The listing builds one solid part. Answer for the finished solid, in the listing's coordinates (mm). Face numbers are marked on the shaded views. A direction names the side the tool comes from. Round coordinates to 2 decimals unless told otherwise and drop trailing zeros. Loops run counter-clockwise (first coordinate to the right, second up) from the corner with the lowest first, then second, coordinate; pieces in that order, holes last. Notation, with made-up numbers: (68.25, -6) -> (113.25, -6) arc R24 ccw to (113.25, 24) -> close; hole circle Ø6 at (-12, 74). An arc over 180 degrees is marked (long way). Answer in a Markdown table with one row per item. Add a question column.
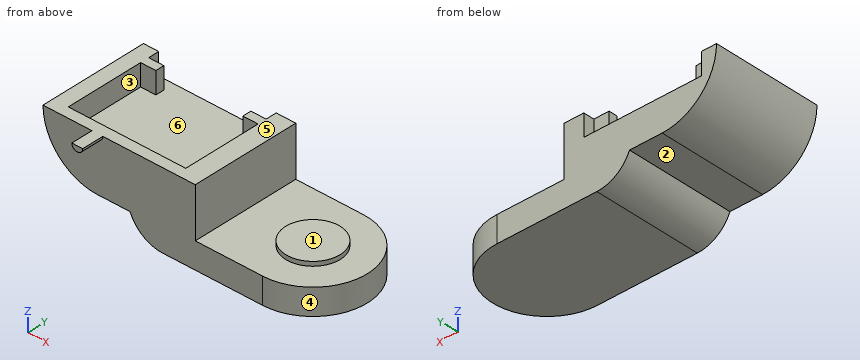
Autodesk Inventor part; units mm, degrees
ref_plane "Work Plane1" through (45, 0, -35) normal (0, 0, -1) x (-1, 0, 0)
ref_plane "YZ Plane" through (0, 0, 0) normal (1, 0, 0) x (0, 1, 0)
ref_plane "XZ Plane" through (0, 0, 0) normal (0, 1, 0) x (-1, 0, 0)
sketch "Sketch1" plane through (0, 0, 0) normal (0, 1, 0) x (-1, 0, 0)
  arc A0 (0, -25) -> (25, 0) centre (0, 0) ccw
  line L0 (25, 0) -> (0, 0) construction
  line L1 (0, -25) -> (0, 0) construction
  arc A1 (25, 0) -> (-25, 0) centre (0, 0) ccw construction
  arc A2 (-25, 0) -> (0, -25) centre (0, 0) ccw construction
  line L2 (18, 10) -> (-36, 10)
  line L3 (-36, 10) -> (-36, -10)
  line L4 (-36, -10) -> (18, -10)
  line L5 (18, -10) -> (18, 10)
  line L6 (11, 10) -> (11, -10)
  line L7 (-29, 10) -> (-29, -10)
  line L8 (0, -25) -> (-45, -25)
  line L9 (-45, -25) -> (-45, 0)
  line L10 (-45, 0) -> (-36, 0)
  line L11 (25, 0) -> (18, 0)
  point P0 (11, 0)
  dimension "d0" = 50
  dimension "d1" = 20
  dimension "d2" = 10
  dimension "d3" = 54
  dimension "d4" = 7
  dimension "d5" = 7
  dimension "d7" = 11
  dimension "d8" = 45
extrude "Extrusion1" add sketch "Sketch1" along normal blind 50 contours L8 L9 L10 L3 L4 L5 L11 A0
sketch "Sketch2" plane through (-18, 0, -10) normal (0, 0, 1) x (1, 0, 0)
  line L0 (7, 50) -> (7, 41) construction
  line L1 (7, 41) -> (0, 41) construction
  line L2 (0, 41) -> (0, 38) construction
  line L3 (0, 0) -> (0, 50) construction
  line L4 (0, 38) -> (7, 38) construction
  line L5 (7, 38) -> (7, 18) construction
  line L6 (7, 18) -> (2, 18) construction
  line L7 (2, 18) -> (2, 15) construction
  line L8 (2, 15) -> (7, 15) construction
  line L9 (7, 15) -> (7, 10) construction
  line L10 (7, 10) -> (47, 10) construction
  line L11 (47, 10) -> (47, 38) construction
  line L12 (47, 38) -> (54, 38) construction
  line L13 (54, 0) -> (54, 50) construction
  line L14 (54, 38) -> (54, 41) construction
  line L15 (54, 41) -> (47, 41) construction
  line L16 (47, 50) -> (20.5, 50) construction
  line L17 (20.5, 50) -> (20.5, 55) construction
  line L18 (20.5, 55) -> (15.5, 55) construction
  line L19 (15.5, 55) -> (15.5, 50) construction
  line L20 (15.5, 50) -> (7, 50) construction
  line L21 (47, 50) -> (47, 41) construction
  line L22 (0, 50) -> (54, 50) construction
  line L23 (7, 41) -> (0, 41)
  line L24 (0, 41) -> (0, 45)
  line L25 (0, 45) -> (7, 45)
  line L26 (7, 45) -> (7, 41)
  line L27 (47, 41) -> (54, 41)
  line L28 (54, 41) -> (54, 45)
  line L29 (54, 45) -> (47, 45)
  line L30 (47, 45) -> (47, 41)
  line L31 (0, 0) -> (0, 50)
  line L32 (0, 5) -> (54, 5)
  line L33 (54, 5) -> (54, 0)
  line L34 (54, 0) -> (0, 0)
  line L35 (0, 0) -> (0, 5)
  point P0 (18, 0)
  point P1 (4.5, 18)
  point P2 (3.5, 38)
  point P3 (18, 55)
  dimension "d11" = 40
  dimension "d12" = 3
  dimension "d13" = 3
  dimension "d16" = 9
  dimension "d17" = 5
  dimension "d18" = 5
  dimension "d19" = 7
  dimension "d20" = 7
  dimension "d21" = 5
  dimension "d22" = 5
  dimension "d23" = 11
  dimension "d24" = 4
  dimension "d29" = 5
extrude "Extrusion2" add sketch "Sketch2" along normal up to surface (10 mm away)
sketch "Sketch4" plane through (0, 0, 0) normal (0, -1, 0) x (1, 0, 0)
  line L0 (-18, 0) -> (36, 0)
  circle A0 centre (0, 0) radius 2.5
  point P0 (2.5, 0)
  point P1 (-2.5, 0)
  dimension "d31" = 5
extrude "Extrusion3" add sketch "Sketch4" along normal blind 10 contours L0 A0 picked at (-0.4734, -0.6858)
sketch "Sketch5" plane through (45, 0, 0) normal (1, 0, 0) x (0, 0, -1)
  line L0 (15, 35) -> (-25, 35)
  line L1 (-25, 35) -> (-25, 15)
  line L2 (-25, 15) -> (15, 15)
  line L3 (15, 15) -> (15, 35)
  line L4 (6, 35) -> (6, 15)
  line L5 (3, 35) -> (3, 15)
  line L6 (-17, 30) -> (-20, 30) construction
  line L7 (-20, 30) -> (-20, 20) construction
  line L8 (-20, 20) -> (-17, 20) construction
  line L9 (-17, 20) -> (-17, 30) construction
  line L10 (0, 5) -> (0, 41)
  line L11 (15, 27.5) -> (20, 27.5)
  line L12 (20, 27.5) -> (20, 22.5)
  line L13 (20, 22.5) -> (15, 22.5)
  line L14 (0, 50) -> (25, 50)
  point P0 (0, 0)
  point P1 (15, 25)
  dimension "d34" = 20
  dimension "d35" = 5
  dimension "d36" = 5
  dimension "d37" = 5
  dimension "d38" = 3
  dimension "d39" = 40
  dimension "d40" = 9
  dimension "d41" = 3
  dimension "d42" = 25
  dimension "d43" = 5
  dimension "d44" = 5
  dimension "d45" = 2.5
  dimension "d48" = 25
ref_plane "Work Plane1" through (45, 0, -35) normal (0, 0, -1) x (-1, 0, 0)
sketch "Sketch6" plane through (45, 0, -35) normal (0, 0, -1) x (-1, 0, 0)
  circle A0 centre (-31, 25) radius 12.5
  circle A1 centre (-31, 25) radius 25
  line L0 (0, 0) -> (0, 50)
  line L1 (0, 25) -> (-26, 25) construction
  line L2 (-31, 50) -> (0, 50)
  line L3 (0, 0) -> (45, 0)
  line L4 (0, 0) -> (-31, 0)
  point P0 (0, 25)
  dimension "d50" = 25
  dimension "d51" = 50
  dimension "d52" = 31
extrude "Extrusion4" add sketch "Sketch6" against normal blind 12 contours A0 | A1 | A1 L2 L0 L4
sketch "Sketch7" plane through (0, 50, 0) normal (0, 1, 0) x (1, 0, 0)
  arc A0 (0, 25) -> (-25, 0) centre (0, 0) ccw
  line L0 (-18, 0) -> (36, 0)
  line L1 (-25, 0) -> (-18, 0)
  line L2 (45, 35) -> (45, 25)
  line L3 (45, 35) -> (30, 35)
  line L4 (45, 25) -> (0, 25)
  arc A1 (30, 35) -> (15, 25) centre (30, 18.75) ccw
  dimension "d56" = 15
  dimension "d59" = 15
  dimension "d60" = 10
extrude "Extrusion5" add sketch "Sketch7" against normal up to surface (50 mm away)
sketch "Sketch8" plane through (45, 0, -23) normal (0, 0, 1) x (1, 0, 0)
  circle A0 centre (31, 25) radius 12.5
  arc A1 (31, 0) -> (31, 50) centre (31, 25) ccw
  point P0 (-45, 0)
  dimension "d63" = 25
extrude "Extrusion6" add sketch "Sketch8" along normal blind 2
equation "\"d59\" = 1.5 * d60"
Item 1: Flat-ended cylindrical pins translate along their axes: P1, Ø3.5, axis at x = -14.5, z = -5.5, coming from the +Y side; P2, Ø1.2, axis at y = 42.5, z = -3, coming from the -X side; P3, Ø2, axis at y = 26, z = -18, coming from the -X side. Find the tip coordinate at first contact, or state that the pin passes through.
Item 2: Consider L1, parallel to X at y = 36.5, z = -4; L2, parallel to Z at x = 79, y = 39; L3, parallel to Y at x = -9, z = -7. Determine where each line is inside the solid, lowest interval first. Write a range as from..to.
Item 3: Section C-C, the plane x = 60.5 is taken. Write down the section's boundary in (y, z).
Item 4: For the marked faces 1, 2 and 3, determine the directions among +Z, -Z, +X, -X, +Y, -Y from which every point of the face is accessible in a straight line to the end or side of a thin tool.
Item 5: Section A-A, the plane y = 25 is taken. Write down the section's boundary in (x, z), and give its area (3 significant figures).
Item 6: Section D-D, the plane y = 39 is taken. Write down the section's boundary in (x, z).
Item 7: Section B-B, the plane z = -8.5 is taken. Write down the section's boundary in (x, y), and give its area (3 significant figures).
Item 8: The mould has two halves that part along Y. Classify the marked faces 4, 5 and 6: +Y half, -Y half, draft (parallel to the pull), parting line (faces both ways), or undercut.
Here are the results:
| question | item | result |
|---|---|---|
| 1 | P1 | stops at y = 45 |
| 1 | P2 | stops at x = -24.88 |
| 1 | P3 | stops at x = -18.33 |
| 2 | L1 | x = -24.68..-18, 36..45 |
| 2 | L2 | z = -35..-23 |
| 2 | L3 | y = 0..5 |
| 3 | outline | (0, -35) -> (50, -35) -> (50, -23) -> (0, -23) -> close |
| 4 | face 1 | +Z, +X, +Y, -Y |
| 4 | face 2 | -Z, -X, +Y, -Y |
| 4 | face 3 | +Z |
| 5 | outline | (-25, 0) arc R25 ccw to (0, -25) -> (15, -25) arc R16.25 ccw to (30, -35) -> (101, -35) -> (101, -23) -> (88.5, -23) -> (88.5, -21) -> (63.5, -21) -> (63.5, -23) -> (45, -23) -> (45, 0) -> (36, 0) -> (36, -10) -> (-18, -10) -> (-18, 0) -> close |
| 5 | area | 2,060 mm² |
| 6 | outline | (-25, 0) arc R25 ccw to (0, -25) -> (15, -25) arc R16.25 ccw to (30, -35) -> (96.71, -35) -> (96.71, -23) -> (45, -23) -> (45, 0) -> (36, 0) -> (36, -10) -> (-18, -10) -> (-18, 0) -> close |
| 7 | outline | (-23.51, 0) -> (45, 0) -> (45, 50) -> (36, 50) -> (36, 45) -> (29, 45) -> (29, 41) -> (36, 41) -> (36, 5) -> (-18, 5) -> (-18, 41) -> (-11, 41) -> (-11, 45) -> (-18, 45) -> (-18, 50) -> (-23.51, 50) -> close |
| 7 | area | 1,050 mm² |
| 8 | face 4 | parting line |
| 8 | face 5 | draft |
| 8 | face 6 | undercut |
